from build123d import *

# Parameters (mm, degrees)
F0_R     = 5.550353
F0_W     = 30.522084
F0_H     = 12.115386
F0_R_2   = 11.169447
F1_DEPTH = 25
F2_DEPTH = 400
F3_W     = 38.587202
F3_H     = 91.675318
F4_DEPTH = 5


with BuildPart() as f1:
    # F0 (on Top) → F1 (new body)
    with BuildSketch(Plane.XY):
        with BuildLine():
            ThreePointArc((28.360015, 93.460975), (25.431083, 100.532043), (18.360015, 103.460975))
            Line((18.360015, 103.460975), (-18.360015, 103.460975))
            ThreePointArc((-18.360015, 103.460975), (-25.431083, 100.532043), (-28.360015, 93.460975))
            Line((-28.360015, 93.460975), (-28.360015, -93.460975))
            ThreePointArc((-28.360015, -93.460975), (-25.431083, -100.532043), (-18.360015, -103.460975))
            Line((-18.360015, -103.460975), (18.360015, -103.460975))
            ThreePointArc((18.360015, -103.460975), (25.431083, -100.532043), (28.360015, -93.460975))
            Line((28.360015, -93.460975), (28.360015, 93.460975))
        make_face()
        with Locations((0, -76.995626)):
            Circle(F0_R, mode=Mode.SUBTRACT)
        with Locations((0, -26.03974)):
            Rectangle(F0_W, F0_H, mode=Mode.SUBTRACT)
        Circle(F0_R_2, mode=Mode.SUBTRACT)
        with Locations((0, 26.03974)):
            Rectangle(F0_W, F0_H, mode=Mode.SUBTRACT)
        with Locations((0, 76.995626)):
            Circle(F0_R, mode=Mode.SUBTRACT)
        with Locations((0, -26.03974)):
            Rectangle(F0_W, F0_H)
        with Locations((0, 26.03974)):
            Rectangle(F0_W, F0_H)
    extrude(amount=F1_DEPTH)

    # F0 (on Top) → F2 (join)
    with BuildSketch(Plane.XY):
        with Locations((0, -26.03974)):
            Rectangle(F0_W, F0_H)
        with Locations((0, 26.03974)):
            Rectangle(F0_W, F0_H)
    extrude(amount=F2_DEPTH)

    # F3 (on face) → F4 (join)
    with BuildSketch(Plane.XY.offset(400)):
        Rectangle(F3_W, F3_H)
    extrude(amount=F4_DEPTH)


solid = f1.part
The listing builds one solid part. Answer for the finished solid, in the listing's coordinates (mm). A direction names the side the tool comes from. Give positions to 0.01 mm unless a question says otherwise; leave off trailing zeros. Order: outer loops, then holes, each group sorted by start corner. A loop starts at its lowest first (then second) coordinate and runs counter-clockwise, first axis right, second up. Notation, with made-up numbers: (74, 21.5) - (78, 21.5) arc R35 cw to (78, 53.5) - close; hole circle Ø8 at (66.25, 38). An arc over 180 degrees is marked (long way). Answer as CSV lines item,"result".
Q1. Which of the six approach directions +Z, -Z, +X, -X, +Y, -Y give full straight-line access (tool end or side, diameter ignored) to faces 4 (the face through (10.654, 3.355, 12.325)), 5 (the face through (0, -19.982, 210)), 6 (the face through (15.261, 26, 210)), 7 (the face through (-15.261, 26, 210)), 8 (the face through (0, 32.097, 210))?
Answer key:
face 4,"-Z"
face 5,"+X, -X"
face 6,"+X, +Y, -Y"
face 7,"-X, +Y, -Y"
face 8,"+X, -X, +Y"
Q2. A cutting plane is placed at B-B, the plane z = 169. Determine the outline of the cut face in (x, y).
Answer key:
outline,"(-15.26, -32.1) - (15.26, -32.1) - (15.26, -19.98) - (-15.26, -19.98) - close; (-15.26, 19.98) - (15.26, 19.98) - (15.26, 32.1) - (-15.26, 32.1) - close"
Q3. Each of these flat-tipped pins is pushed along its axis until it touches: pin 1 Ø6 at (x, z) = (-9, 282) entering from +Y; pin 2 Ø4 at (x, z) = (-1, 401.5) entering from +Y; pin 3 Ø4 at (y, z) = (-13.5, 403.5) entering from -X. Where does it stop, or does it pass through?
Answer key:
pin 1,"stops at y = 32.1"
pin 2,"stops at y = 45.84"
pin 3,"stops at x = -19.29"
Q4. A cutting plane is placed at C-C, the plane x = 0. Determine the outline of the cut face in (y, z).
Answer key:
outline,"(-103.46, 0) - (-82.55, 0) - (-82.55, 25) - (-103.46, 25) - close; (-71.45, 0) - (-11.17, 0) - (-11.17, 25) - (-19.98, 25) - (-19.98, 400) - (19.98, 400) - (19.98, 25) - (11.17, 25) - (11.17, 0) - (71.45, 0) - (71.45, 25) - (32.1, 25) - (32.1, 400) - (45.84, 400) - (45.84, 405) - (-45.84, 405) - (-45.84, 400) - (-32.1, 400) - (-32.1, 25) - (-71.45, 25) - close; (82.55, 0) - (103.46, 0) - (103.46, 25) - (82.55, 25) - close"
Q5. Determine the mould class of faces 1 (the face through (0, 19.982, 210)), 2 (the face through (0, -32.097, 210)), 3 (the face through (-28.36, 1, 12)) for opening direction Y: pulls with the +Y half, pulls with the -Y half, needs draft (parallel to the pull), parting line crosses it, or undercut.
Answer key:
face 1,"undercut"
face 2,"pulls with the -Y half"
face 3,"needs draft"
Q6. A cutting plane is placed at A-A, the plane y = 0. Determine the outline of the cut face in (x, z).
Answer key:
outline,"(-28.36, 0) - (-11.17, 0) - (-11.17, 25) - (-28.36, 25) - close; (-19.29, 400) - (19.29, 400) - (19.29, 405) - (-19.29, 405) - close; (11.17, 0) - (28.36, 0) - (28.36, 25) - (11.17, 25) - close"
Q7. Straight lines are drawn through the part: L1, parallel to Y at x = 0, z = 10; L2, parallel to Z at x = 13, y = 36.5; L3, parallel to Z at x = -12.5, y = -93. For each, find the intervals that lie inside material, in ascending order.
Answer key:
L1,"y = -103.46 to -82.55, -71.45 to -11.17, 11.17 to 71.45, 82.55 to 103.46"
L2,"z = 0 to 25, 400 to 405"
L3,"z = 0 to 25"
